Could you check a few things on this model? Use its own coordinates, in mm. A direction names the side the tool comes from. Coordinates: 2 decimals unless noted, no trailing zeros. Write each loop counter-clockwise with the first axis right and the second up, starting at its lowest first coordinate (ties: lowest second). Pieces come first, ordered by that corner, then holes.
```python
from build123d import *

# Parameters (mm, degrees)
F1_DEPTH      = 14
F1_DEPTH_BACK = 14
F2_R          = 5.401545
F3_DEPTH      = 100


with BuildPart() as f1:
    # F0 (on Top) → F1 (new body, two sides)
    with BuildSketch(Plane.XY) as f1_sk:
        with BuildLine():
            ThreePointArc((-22.312058, -1.975505), (-20.700792, -1.520545), (-20, 0))
            ThreePointArc((-20, 0), (-20.700792, 1.520545), (-22.312058, 1.975505))
            ThreePointArc((-22.312058, 1.975505), (-24, 0), (-22.312058, -1.975505))
        make_face()
        with BuildLine():
            ThreePointArc((-22.312058, 1.975505), (-20.700792, 1.520545), (-20, 0))
            ThreePointArc((-20, 0), (-20.700792, -1.520545), (-22.312058, -1.975505))
            Line((-22.312058, -1.975505), (-1.695299, -5.232204))
            ThreePointArc((-1.695299, -5.232204), (-5.5, 0), (-1.695299, 5.232204))
            Line((-1.695299, 5.232204), (-22.312058, 1.975505))
        make_face()
        with BuildLine():
            Line((0, 5.5), (-1.695299, 5.232204))
            ThreePointArc((-1.695299, 5.232204), (-5.5, 0), (-1.695299, -5.232204))
            Line((-1.695299, -5.232204), (0, -5.5))
            ThreePointArc((0, -5.5), (3.889087, -3.889087), (5.5, 0))
            ThreePointArc((5.5, 0), (3.889087, 3.889087), (0, 5.5))
        make_face()
        with BuildLine():
            ThreePointArc((0, 5.5), (-0.85816, 5.432639), (-1.695299, 5.232204))
            Line((-1.695299, 5.232204), (0, 5.5))
        make_face()
        with BuildLine():
            Line((0, -5.5), (-1.695299, -5.232204))
            ThreePointArc((-1.695299, -5.232204), (-0.85816, -5.432639), (0, -5.5))
        make_face()
    extrude(amount=F1_DEPTH)
    extrude(f1_sk.sketch, amount=-F1_DEPTH_BACK)

    # F2 (on Right) → F3 (join)
    with BuildSketch(Plane.YZ):
        Circle(F2_R)
    extrude(amount=F3_DEPTH)


solid = f1.part
```
1. I want a section at A-A on z = 0. Please give me the cut outline in (x, y).
Verdict:
outline: (-22.31, -1.98) - (-1.7, -5.23) arc R5.5 ccw to (0, -5.5) arc R5.5 ccw to (1.04, -5.4) - (100, -5.4) - (100, 5.4) - (1.04, 5.4) arc R5.5 ccw to (0, 5.5) arc R5.5 ccw to (-1.7, 5.23) - (-22.31, 1.98) arc R2 ccw to start
2. For pin 1 (5 mm diameter, centred on x = 60.5, y = -3, fed in from +Z); pin 2 (5 mm diameter, centred on x = 4.5, z = -4, fed in from -Y); pin 3 (2 mm diameter, centred on y = 0.5, z = 8, fed in from +X), each with a flat end and sliding along its axis, tell me the tip position at first contact or that it passes through.
Verdict:
pin 1: stops at z = 5.38
pin 2: stops at y = -5.19
pin 3: stops at x = 5.5
3. I want a section at C-C on x = 35. Please give me the cut outline in (y, z), plus the area to 3 significant figures.
Verdict:
outline: circle Ø10.8 at (0, 0)
area: 91.7 mm2
4. Please list where these lines run through material, in increasing order: line 1 along X through (y, z) = (0, -12.5); line 2 along Z through (x, y) = (79.5, -1.25); line 3 along Z through (x, y) = (64, -4.5).
Verdict:
line 1: x = -24 to 5.5
line 2: z = -5.25 to 5.25
line 3: z = -2.99 to 2.99
5. I want a section at D-D on z = 9.75. Please give me the cut outline in (x, y), plus the area to 3 significant figures.
Verdict:
outline: (-22.31, -1.98) - (-1.7, -5.23) arc R5.5 ccw to (0, -5.5) arc R5.5 ccw to (5.5, 0) arc R5.5 ccw to (0, 5.5) arc R5.5 ccw to (-1.7, 5.23) - (-22.31, 1.98) arc R2 ccw to start
area: 220 mm2
6. On a 3-axis mill with a long thin cutter (end or side, diameter ignored), from which of +Z, -Z, +X, -X, +Y, -Y can I reach the whole of each face in a straight line? I mean faces 1 (the face through (49.82, -1.171, -5.273)), 2 (the face through (-12.15, -3.58, 0.2)). Say none if no direction works.
Verdict:
face 1: +X
face 2: +Z, -Z, -X, -Y
7. I want a section at B-B on y = 3.5. Please give me the cut outline in (x, z).
Verdict:
outline: (-12.66, -14) - (4.24, -14) - (4.24, -4.11) - (100, -4.11) - (100, 4.11) - (4.24, 4.11) - (4.24, 14) - (-12.66, 14) - close
